from build123d import *

# Parameters (mm, degrees)
SKETCH1_R           = 37
SKETCH1_R_2         = 2.75
BOSS_EXTRUDE1_DEPTH = 2
SKETCH2_R           = 37
SKETCH2_R_2         = 30
BOSS_EXTRUDE2_DEPTH = 3.5


with BuildPart() as part:
    # Sketch1 → Boss-Extrude1 (new body)
    with BuildSketch(Plane(origin=(0, 0, 0), x_dir=(1, 0, 0), z_dir=(0, 1, 0))):
        Circle(SKETCH1_R)
        with Locations((0, 16.57)):
            Circle(SKETCH1_R_2, mode=Mode.SUBTRACT)
        with Locations((-14.350040941, 8.285)):
            Circle(SKETCH1_R_2, mode=Mode.SUBTRACT)
        with Locations((-14.350040941, -8.285)):
            Circle(SKETCH1_R_2, mode=Mode.SUBTRACT)
        with Locations((0, -16.57)):
            Circle(SKETCH1_R_2, mode=Mode.SUBTRACT)
        with Locations((14.350040941, -8.285)):
            Circle(SKETCH1_R_2, mode=Mode.SUBTRACT)
        with Locations((14.350040941, 8.285)):
            Circle(SKETCH1_R_2, mode=Mode.SUBTRACT)
    extrude(amount=BOSS_EXTRUDE1_DEPTH)

    # Sketch2 → Boss-Extrude2 (add)
    with BuildSketch(Plane(origin=(0, 2, 0), x_dir=(1, 0, 0), z_dir=(0, 1, 0))):
        Circle(SKETCH2_R)
        Circle(SKETCH2_R_2, mode=Mode.SUBTRACT)
    extrude(amount=BOSS_EXTRUDE2_DEPTH)


solid = part.part
The model under review builds one solid part; all positions refer to its coordinate system, in mm. A direction names the side the tool comes from. Round coordinates to 2 decimals unless told otherwise and drop trailing zeros. Write each loop counter-clockwise with the first axis right and the second up, starting at its lowest first coordinate (ties: lowest second). Pieces come first, ordered by that corner, then holes. Notation, with made-up numbers: (15, 88) - (54, 88) arc R15 ccw to (54, 107) - close; hole circle Ø5 at (-4, 40.25). An arc over 180 degrees is marked (long way). One line per item, written item: value. Start each with the question number.
1. Consider section B-B on z = 0. Write out the cut boundary in (x, y), and give its area (3 significant figures).
2. To check wall thickness, follow L1, parallel to Z at x = 0, y = 1.3; L2, parallel to X at y = 4.3, z = 0; L3, parallel to Y at x = -11.5, z = 0. State the ranges of each line that lie inside material, in increasing order. Write a range as from..to.
3. Consider section C-C on x = -23.5. Write out the cut boundary in (y, z).
4. Consider section A-A on x = 0. Write out the cut boundary in (y, z), and give its area (3 significant figures).
5. Consider section D-D on z = 16.57. Write out the cut boundary in (x, y), and give its area (3 significant figures).
6. Clearance check with flat-ended pins moving along their axes: P1, Ø1.5, axis at y = 3.5, z = 2.5, coming from the -X side; P2, Ø2, axis at x = -4, y = 4.5, coming from the +Z side; P3, Ø1, axis at y = 5, z = 14.5, coming from the +X side. State where each tip first meets the part, or that it passes through.
7. Machinability: for faces 1 (the face through (-29.97, 3.73, -1.32)), 2 (the face through (-0.358, 0.986, 13.843)), which of the approach directions +Z, -Z, +X, -X, +Y, -Y give a long, thin tool a straight path to every point of the face, cutting with its end or side? Answer none if there is none.
8. The part is to be moulded in two halves that separate along X. For faces 3 (the face through (-11.727, 0.986, 7.459)), 4 (the face through (-8.02, 2.71, 36.12)), 5 (the face through (-0.2, 5.5, -30.3)), say which applies: released by +X, released by -X, zero draft, split by the parting line, or undercut.
Checks:
1. outline: (-37, 0) - (37, 0) - (37, 5.5) - (30, 5.5) - (30, 2) - (-30, 2) - (-30, 5.5) - (-37, 5.5) - close
1. area: 197 mm^2
2. L1: z = -37..-19.32, -13.82..13.82, 19.32..37
2. L2: x = -37..-30, 30..37
2. L3: y = 0..2
3. outline: (0, -28.58) - (5.5, -28.58) - (5.5, -18.65) - (2, -18.65) - (2, 18.65) - (5.5, 18.65) - (5.5, 28.58) - (0, 28.58) - close
4. outline: (0, -37) - (5.5, -37) - (5.5, -30) - (2, -30) - (2, -19.32) - (0, -19.32) - close; (0, -13.82) - (2, -13.82) - (2, 13.82) - (0, 13.82) - close; (0, 19.32) - (2, 19.32) - (2, 30) - (5.5, 30) - (5.5, 37) - (0, 37) - close
4. area: 175 mm^2
5. outline: (-33.08, 0) - (-2.75, 0) - (-2.75, 2) - (-25.01, 2) - (-25.01, 5.5) - (-33.08, 5.5) - close; (2.75, 0) - (33.08, 0) - (33.08, 5.5) - (25.01, 5.5) - (25.01, 2) - (2.75, 2) - close
5. area: 178 mm^2
6. P1: stops at x = -36.96
6. P2: stops at z = 36.88
6. P3: stops at x = 34.25
7. face 1: +Y
7. face 2: +Y, -Y
8. face 3: undercut
8. face 4: split by the parting line
8. face 5: zero draft
